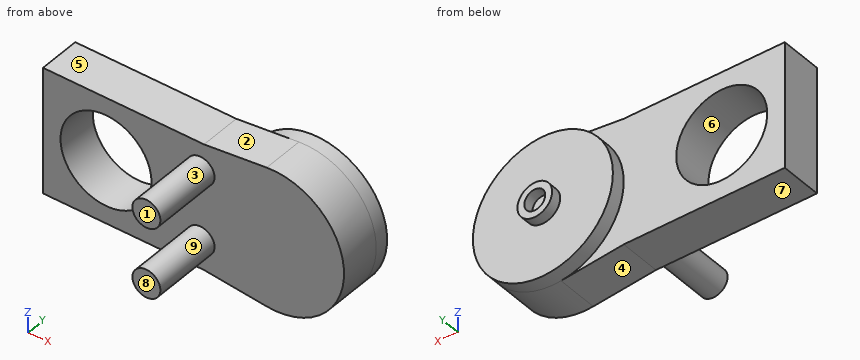
```python
from build123d import *

# Parameters (mm, degrees)
BOSS_EXTRUDE2_OUTLINE_R = 6.5
BOSS_EXTRUDE2_DEPTH     = 5.95
SKETCH3_R               = 10
BOSS_EXTRUDE3_DEPTH     = 2
SKETCH4_R               = 2
BOSS_EXTRUDE4_DEPTH     = 10
SKETCH5_R               = 2.475
SKETCH5_R_2             = 1.5
BOSS_EXTRUDE5_DEPTH     = 1.5


# Read off the part's stored shape, not the designer's step: Boss-Extrude2
with BuildPart() as part:
    # Boss-Extrude2 outline → Boss-Extrude2 (new body)
    with BuildSketch(Plane(origin=(0, 0, 0), x_dir=(1, 0, 0), z_dir=(0, 1, 0))):
        with BuildLine():
            Line((14, 9), (-9, 9))
            Line((-9, 9), (-9, -9))
            Line((-9, -9), (14, -9))
            Line((14, -9), (22.950276243, -9.944751381))
            ThreePointArc((22.950276243, -9.944751381), (34, 0), (22.950276243, 9.944751381))
            Line((22.950276243, 9.944751381), (14, 9))
        make_face()
        Circle(BOSS_EXTRUDE2_OUTLINE_R, mode=Mode.SUBTRACT)
    extrude(amount=BOSS_EXTRUDE2_DEPTH)

    # Sketch3 → Boss-Extrude3 (add)
    with BuildSketch(Plane(origin=(0, 5.95, 0), x_dir=(1, 0, 0), z_dir=(0, 1, 0))):
        with Locations(Location((24, 0, 0), (0, 0, 96.025575008))):
            Circle(SKETCH3_R)
    extrude(amount=BOSS_EXTRUDE3_DEPTH)

    # Sketch4 → Boss-Extrude4 (add)
    with BuildSketch(Plane.XZ):
        with Locations(Location((13.5, 5, 0), (0, 0, 90))):
            Circle(SKETCH4_R)
        with Locations(Location((13.5, -5, 0), (0, 0, 90))):
            Circle(SKETCH4_R)
    extrude(amount=BOSS_EXTRUDE4_DEPTH)

    # Sketch5 → Boss-Extrude5 (add)
    with BuildSketch(Plane(origin=(0, 7.95, 0), x_dir=(1, 0, 0), z_dir=(0, 1, 0))):
        with Locations(Location((24, 0, 0), (0, 0, 270))):
            Circle(SKETCH5_R)
        with Locations(Location((24, 0, 0), (0, 0, 270))):
            Circle(SKETCH5_R_2, mode=Mode.SUBTRACT)
    extrude(amount=BOSS_EXTRUDE5_DEPTH)


solid = part.part
```
Geometry check sheet. Reference: the model listing, model coordinates, mm. Face numbers are marked on the shaded views. A direction names the side the tool comes from. Give positions to 0.01 mm unless a question says otherwise; leave off trailing zeros. Loops run counter-clockwise (first coordinate to the right, second up) from the corner with the lowest first, then second, coordinate; pieces in that order, holes last. Notation, with made-up numbers: M 24.25,59 L 72.25,59 A33 ccw 72.25,97 Z; hole C -39,28.25 d7. An arc over 180 degrees is marked long. Write item = value, one per line. Start each with the question number.
1. Draft check along Z on the marked faces 1, 2, 3 and 4. Enter one of: +Z half, -Z half, draft (parallel to the pull), parting line (faces both ways), or undercut.
2. Tool access check on the marked faces 5, 6, 7, 8 and 9. Record the directions out of +Z, -Z, +X, -X, +Y, -Y that give a thin tool (end or side, any length) a straight path to the whole face; none if there is none.
3. Thickness scan on probe 1 along Z at (x, y) = (0, 3.85); probe 2 along X at (y, z) = (9.15, 0) (3 decimals); probe 3 along Z at (x, y) = (13.5, -7.25). Record the ranges inside material, lowest first.
4. Go/stop test with flat-tipped pins: P1, Ø1, axis at x = 22.5, z = 2, coming from the +Y side; P2, Ø6.5, axis at x = 5.5, y = 4, coming from the +Z side; P3, Ø2, axis at x = 28, z = 0.5, coming from the -Y side; P4, Ø3, axis at x = 7, y = 2, coming from the -Z side. Record where each tip stops, or that it passes through.
5. Section check A-A, the plane z = 0. Enter the section's corners in (x, y) (3 decimals).
6. Section check B-B, the plane x = 0. Enter the section's corners in (y, z).
7. Section check C-C, the plane y = 2.5. Enter the section's corners in (x, z).
8. Section check D-D, the plane x = 13.5. Enter the section's corners in (y, z), plus the area to 3 significant figures.
Values follow:
q1.face_1 = draft
q1.face_2 = +Z half
q1.face_3 = undercut
q1.face_4 = -Z half
q2.face_5 = +Z, -X, +Y, -Y
q2.face_6 = +Y, -Y
q2.face_7 = -Z, -X, +Y, -Y
q2.face_8 = +Z, -Z, +X, -X, -Y
q2.face_9 = -Y
q3.probe_1 = -9 to -6.5, 6.5 to 9
q3.probe_2 = 21.525 to 22.5, 25.5 to 26.475
q3.probe_3 = -7 to -3, 3 to 7
q4.P1 = 9.45
q4.P2 = 9
q4.P3 = 0
q4.P4 = -9
q5.outline = M -9,0 L -6.5,0 L -6.5,5.95 L -9,5.95 Z; M 6.5,0 L 34,0 L 34,7.95 L 26.475,7.95 L 26.475,9.45 L 25.5,9.45 L 25.5,7.95 L 22.5,7.95 L 22.5,9.45 L 21.525,9.45 L 21.525,7.95 L 14,7.95 L 14,5.95 L 6.5,5.95 Z
q6.outline = M 0,-9 L 5.95,-9 L 5.95,-6.5 L 0,-6.5 Z; M 0,6.5 L 5.95,6.5 L 5.95,9 L 0,9 Z
q7.outline = M -9,-9 L 14,-9 L 22.95,-9.94 A10 ccw long 22.95,9.94 L 14,9 L -9,9 Z; hole C 0,0 d13
q8.outline = M -10,-7 L 0,-7 L 0,-9 L 5.95,-9 L 5.95,9 L 0,9 L 0,7 L -10,7 L -10,3 L 0,3 L 0,-3 L -10,-3 Z
q8.area = 187 mm^2
